Could you check a few things on this model? Use its own coordinates, in mm. Face numbers are marked on the shaded views. A direction names the side the tool comes from. Give positions to 0.01 mm unless a question says otherwise; leave off trailing zeros. Order: outer loops, then holes, each group sorted by start corner. A loop starts at its lowest first (then second) coordinate and runs counter-clockwise, first axis right, second up.
(1) Imagine slicing it at D-D, the plane y = -32. Write out the boundary of the cut face in (x, z).
(2) If I drill on probe 1 along Z at (x, y) = (7, -9); probe 2 along Z at (x, y) = (69.5, -44.5); probe 3 along X at (y, z) = (-13, -32), over which ranges is the centre line in solid material (lowest first)?
(3) Imagine slicing it at B-B, the plane y = -42. Write out the boundary of the cut face in (x, z), then the cut area to 3 significant figures.
(4) Imagine slicing it at C-C, the plane z = -31.5. Write out the boundary of the cut face in (x, y), then the cut area to 3 significant figures.
(5) Will these pins go through, and if not, where does the flat tip stop? pin 1 (3.5 mm diameter, centred on x = -6.42, y = 2.78, fed in from +Z); pin 2 (2 mm diameter, centred on x = 6.42, y = -2.78, fed in from -Z); pin 3 (25 mm diameter, centred on x = 49.5, y = -25.5, fed in from -Z); pin 4 (1.5 mm diameter, centred on y = -12.5, z = -15.5, fed in from +X).
(6) If we mould it in two halves opening along Z, with no side actions, what happens to the marked faces 1, 2 and 3? For each: released by +Z, released by -Z, zero draft, split by the parting line, or undercut.
(7) On a 3-axis mill with a long thin cutter (end or side, diameter ignored), from which of +Z, -Z, +X, -X, +Y, -Y can I reach the whole of each face in a straight line? I mean the marked faces 4 and 5. Say none if no direction works.
(8) Imagine slicing it at A-A, the plane x = 0. Write out the boundary of the cut face in (y, z).
from build123d import *

# Parameters (mm, degrees)
ESQUISSE2_R        = 1.275
ESQUISSE2_R_2      = 3
BOSS_EXTRU_1_DEPTH = 3
BOSS_EXTRU_4_DEPTH = 51
CONG_1_R           = 2
ESQUISSE6_R        = 1.275
BOSS_EXTRU_5_DEPTH = 3
CONG_2_R           = 2


with BuildPart() as part:
    # Esquisse2 → Boss.-Extru.1 (new body)
    with BuildSketch(Plane.XY.offset(-10.755524)):
        with BuildLine():
            Line((42.518708, -7.493961), (3.9696, 9.178359))
            ThreePointArc((3.9696, 9.178359), (-9.178359, 3.9696), (-3.9696, -9.178359))
            Line((-3.9696, -9.178359), (34.579508, -25.850679))
            Line((34.579508, -25.850679), (32.594708, -30.439859))
            Line((32.594708, -30.439859), (78.486504, -50.287859))
            Line((78.486504, -50.287859), (90.395304, -22.752781))
            Line((90.395304, -22.752781), (44.503508, -2.904781))
            Line((44.503508, -2.904781), (42.518708, -7.493961))
        make_face()
        with Locations((6.424851, -2.77872)):
            Circle(ESQUISSE2_R, mode=Mode.SUBTRACT)
        with Locations((-2.77872, -6.424851)):
            Circle(ESQUISSE2_R, mode=Mode.SUBTRACT)
        with Locations((-6.424851, 2.77872)):
            Circle(ESQUISSE2_R, mode=Mode.SUBTRACT)
        with Locations((2.77872, 6.424851)):
            Circle(ESQUISSE2_R, mode=Mode.SUBTRACT)
        with Locations((75.882124, -43.713879)):
            Circle(ESQUISSE2_R_2, mode=Mode.SUBTRACT)
        with Locations((83.821324, -25.357161)):
            Circle(ESQUISSE2_R_2, mode=Mode.SUBTRACT)
        with Locations((47.107888, -9.478761)):
            Circle(ESQUISSE2_R_2, mode=Mode.SUBTRACT)
        with Locations((39.168688, -27.835479)):
            Circle(ESQUISSE2_R_2, mode=Mode.SUBTRACT)
    extrude(amount=BOSS_EXTRU_1_DEPTH)

    # Esquisse5 → Boss.-Extru.4 (add)
    with BuildSketch(Plane(origin=(0, 0, -10.755524), x_dir=(-1, 0, 0), z_dir=(0, 0, -1))):
        Polygon((-13.469282, -16.720599), (-21.408482, 1.636119), (-23.244154, 0.842199), (-15.304954, -17.514519), align=None)
    extrude(amount=BOSS_EXTRU_4_DEPTH)

    # Congé1
    cong_1_edges = [part.edges().sort_by_distance(p)[0] for p in [
        (19.274554, -8.33616, -10.755524),
        (17.438882, -7.54224, -10.755524),
    ]]
    fillet(cong_1_edges, radius=CONG_1_R)

    # Esquisse6 → Boss.-Extru.5 (add)
    with BuildSketch(Plane(origin=(0, 0, -61.755524), x_dir=(-1, 0, 0), z_dir=(0, 0, -1))):
        with BuildLine():
            Line((3.9696, -9.178359), (-11.63361, -15.926679))
            Line((-11.63361, -15.926679), (-15.304954, -17.514519))
            Line((-15.304954, -17.514519), (-23.244154, 0.842199))
            Line((-23.244154, 0.842199), (-19.57281, 2.430039))
            Line((-19.57281, 2.430039), (-3.9696, 9.178359))
            ThreePointArc((-3.9696, 9.178359), (9.178359, 3.9696), (3.9696, -9.178359))
        make_face()
        with Locations((6.424851, 2.77872)):
            Circle(ESQUISSE6_R, mode=Mode.SUBTRACT)
        with Locations((-2.77872, 6.424851)):
            Circle(ESQUISSE6_R, mode=Mode.SUBTRACT)
        with Locations((-6.424851, -2.77872)):
            Circle(ESQUISSE6_R, mode=Mode.SUBTRACT)
        with Locations((2.77872, -6.424851)):
            Circle(ESQUISSE6_R, mode=Mode.SUBTRACT)
    extrude(amount=BOSS_EXTRU_5_DEPTH)

    # Congé2
    cong_2_edges = [part.edges().sort_by_distance(p)[0] for p in [
        (17.438882, -7.54224, -61.755524),
        (19.274554, -8.33616, -64.755524),
    ]]
    fillet(cong_2_edges, radius=CONG_2_R)


solid = part.part
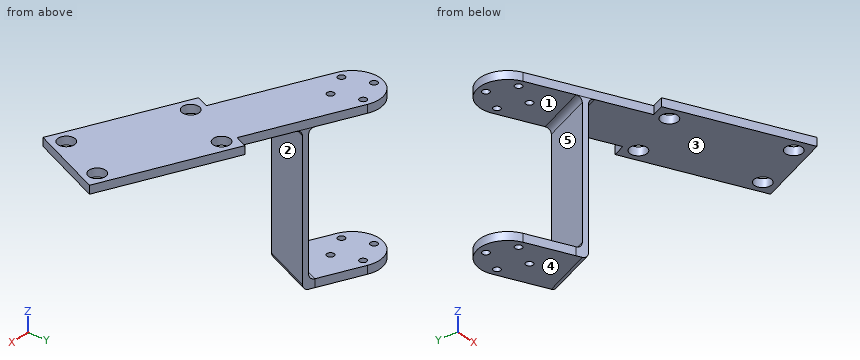
Answer block:
1. outline: (36.2, -10.76) - (86.4, -10.76) - (86.4, -7.76) - (36.2, -7.76) - close
2. probe 1: z = -64.76 to -61.76, -10.76 to -7.76
2. probe 2: z = -10.76 to -7.76
2. probe 3: x = 15.08 to 17.26
3. outline: (59.32, -10.76) - (73.42, -10.76) - (73.42, -7.76) - (59.32, -7.76) - close; (78.34, -10.76) - (82.07, -10.76) - (82.07, -7.76) - (78.34, -7.76) - close
3. area: 53.5 mm2
4. outline: (13.47, -16.72) - (15.3, -17.51) - (23.24, 0.84) - (21.41, 1.64) - close
4. area: 40.0 mm2
5. pin 1: stops at z = -7.76
5. pin 2: passes through
5. pin 3: stops at z = -10.76
5. pin 4: stops at x = 17.8
6. face 1: undercut
6. face 2: zero draft
6. face 3: released by -Z
7. face 4: -Z, +X, -X, +Y, -Y
7. face 5: -X, +Y
8. outline: (-10.9, -64.76) - (10, -64.76) - (10, -61.76) - (-10.9, -61.76) - close; (-10.9, -10.76) - (10, -10.76) - (10, -7.76) - (-10.9, -7.76) - close
